Verification items for this drawing (mm, ordinates from the low corner). A direction names the side the tool comes from. Give positions to 0.01 mm unless a question says otherwise; leave off trailing zeros. Loops run counter-clockwise (first coordinate to the right, second up) from the corner with the lowest first, then second, coordinate; pieces in that order, holes last. Notation, with made-up numbers: M 55,-14.75 L 97,-14.75 A27 cw 97,15.25 Z; hole C 70,-18 d8. An arc over 180 degrees is marked long. Use a Markdown table: item, result.
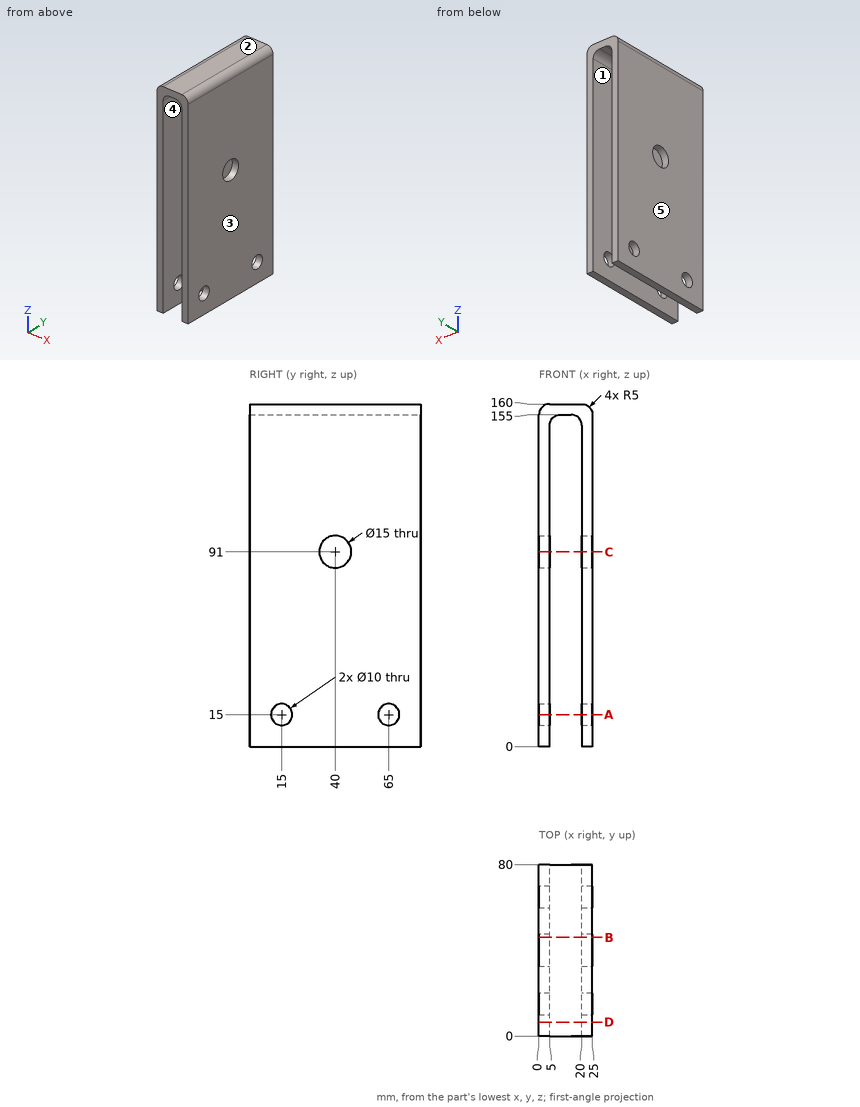
(1) Material ranges on line 1 (X direction, y = 70, z = 116); line 2 (Z direction, x = 12, y = 53); line 3 (Z direction, x = 1.5, y = 40), recorded low to high.
Results below:
| item | result |
|---|---|
| line 1 | 0 to 5, 20 to 25 |
| line 2 | 155 to 160 |
| line 3 | 0 to 83.5, 98.5 to 158.57 |
(2) Draft check along X on the marked faces 1, 2 and 3. Enter one of: +X half, -X half, draft (parallel to the pull), parting line (faces both ways), or undercut.
Results below:
| item | result |
|---|---|
| face 1 | undercut |
| face 2 | draft |
| face 3 | +X half |
(3) Gauge pin test, flat ends, axial feed: P1, Ø9, axis at y = 40, z = 91, coming from the +X side; P2, Ø2.5, axis at x = 13, y = 51.5, coming from the -Z side. Record the tip position at first contact, or that the pin passes through.
Results below:
| item | result |
|---|---|
| P1 | through |
| P2 | z = 155 |
(4) Cross-section at A-A on z = 15. Record the cut outline in (x, y).
Results below:
| item | result |
|---|---|
| outline | M 0,0 L 5,0 L 5,10 L 0,10 Z; M 0,20 L 5,20 L 5,60 L 0,60 Z; M 0,70 L 5,70 L 5,80 L 0,80 Z; M 20,0 L 25,0 L 25,10 L 20,10 Z; M 20,20 L 25,20 L 25,60 L 20,60 Z; M 20,70 L 25,70 L 25,80 L 20,80 Z |
(5) Cross-section at C-C on z = 91. Record the cut outline in (x, y), then the cut area to 3 significant figures.
Results below:
| item | result |
|---|---|
| outline | M 0,0 L 5,0 L 5,32.5 L 0,32.5 Z; M 0,47.5 L 5,47.5 L 5,80 L 0,80 Z; M 20,0 L 25,0 L 25,32.5 L 20,32.5 Z; M 20,47.5 L 25,47.5 L 25,80 L 20,80 Z |
| area | 650 mm^2 |
(6) Cross-section at B-B on y = 46. Record the cut outline in (x, z).
Results below:
| item | result |
|---|---|
| outline | M 0,0 L 5,0 L 5,86.5 L 0,86.5 Z; M 0,95.5 L 5,95.5 L 5,150 A5 cw 10,155 L 15,155 A5 cw 20,150 L 20,95.5 L 25,95.5 L 25,155 A5 ccw 20,160 L 5,160 A5 ccw 0,155 Z; M 20,0 L 25,0 L 25,86.5 L 20,86.5 Z |
(7) Cross-section at D-D on y = 6.5. Record the cut outline in (x, z), then the cut area to 4 significant figures.
Results below:
| item | result |
|---|---|
| outline | M 0,0 L 5,0 L 5,150 A5 cw 10,155 L 15,155 A5 cw 20,150 L 20,0 L 25,0 L 25,155 A5 ccw 20,160 L 5,160 A5 ccw 0,155 Z |
| area | 1,675 mm^2 |
(8) Set-up check for the marked faces 4 and 5: record each of +Z, -Z, +X, -X, +Y, -Y from which the full face is reachable in a straight line by a thin tool's end or side.
Results below:
| item | result |
|---|---|
| face 4 | -Z, +Y, -Y |
| face 5 | +Z, -Z, -X, +Y, -Y |
